from build123d import *

# Parameters (mm, degrees)
SKETCH2_W           = 25.4
SKETCH2_H           = 241.3
BOSS_EXTRUDE1_DEPTH = 0.79375


with BuildPart() as part:
    # Sketch2 → Boss-Extrude1 (new, symmetric)
    with BuildSketch(Plane.XY):
        with BuildLine():
            ThreePointArc((0, -50.8), (35.921024484, -35.921024484), (50.8, 0))
            Line((50.8, 0), (182.88, 0))
            Line((182.88, 0), (182.88, -241.3))
            Line((182.88, -241.3), (0, -241.3))
            Line((0, -241.3), (0, -50.8))
        make_face()
        with Locations((195.58, -120.65)):
            Rectangle(SKETCH2_W, SKETCH2_H)
    extrude(amount=BOSS_EXTRUDE1_DEPTH, both=True)


solid = part.part
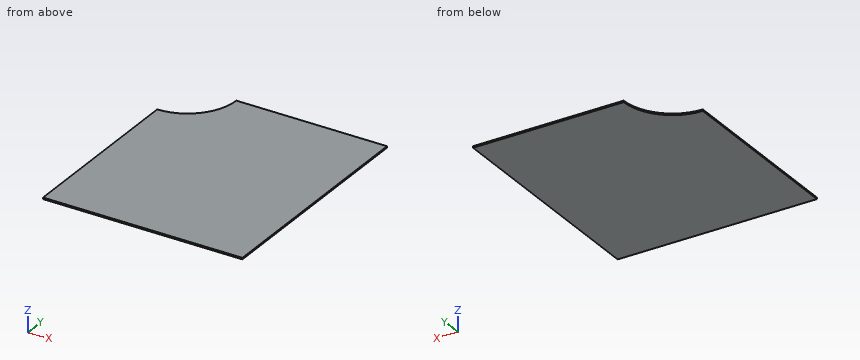
Part model, mm, in its own coordinate system. Coordinates: 2 decimals unless noted, no trailing zeros. Write each loop counter-clockwise with the first axis right and the second up, starting at its lowest first coordinate (ties: lowest second). Pieces come first, ordered by that corner, then holes. Notation, with made-up numbers: M 59,61.5 L 85,61.5 A9 ccw 85,70.5 Z; hole C 42,41.5 d8. An arc over 180 degrees is marked long. Return JSON: item names as keys, results as strings.
1. Saw through at C-C, the plane x = 30.5. Write the cut outline in (y, z) (3 decimals).
Determined:
{"outline": "M -241.3,-0.794 L -40.625,-0.794 L -40.625,0.794 L -241.3,0.794 Z"}
2. Probe L1, parallel to Y at x = 15.5, z = -0.15; L2, parallel to Y at x = 10.5, z = 0.6. List the from-to ranges inside material, lowest first.
Determined:
{"L1": "-241.3 to -48.38", "L2": "-241.3 to -49.7"}
3. Saw through at B-B, the plane y = -27. Write the cut outline in (x, z).
Determined:
{"outline": "M 43.03,-0.79 L 208.28,-0.79 L 208.28,0.79 L 43.03,0.79 Z"}
4. Saw through at A-A, the plane z = 0.3. Write the cut outline in (x, y), then the cut area to 3 significant figures.
Determined:
{"outline": "M 0,-241.3 L 208.28,-241.3 L 208.28,0 L 50.8,0 A50.8 cw 0,-50.8 Z", "area": "48,200 mm²"}
